Geometry check sheet. Reference: the model listing, model coordinates, mm. Face numbers are marked on the shaded views. A direction names the side the tool comes from. Coordinates: 2 decimals unless noted, no trailing zeros. Write each loop counter-clockwise with the first axis right and the second up, starting at its lowest first coordinate (ties: lowest second). Pieces come first, ordered by that corner, then holes. Notation, with made-up numbers: M 52.25,-12 L 66.25,-12 A7 cw 66.25,-3 Z; hole C 8,-24 d8. An arc over 180 degrees is marked long. Answer as a JSON object with one key per item and string values. Group by question number.
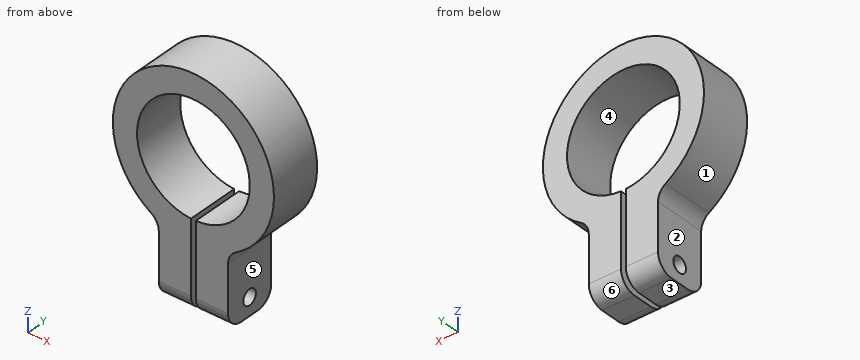
```python
from build123d import *

# Parameters (mm, degrees)
F1_DEPTH = 6.5
F2_R     = 0.95
F3_DEPTH = 25
F4_R     = 2
F5_R     = 2


with BuildPart() as f1:
    # F0 (on Front) → F1 (new body)
    with BuildSketch(Plane.XZ):
        with BuildLine():
            Line((4.29925, -18.028646), (4.29925, -9.028646))
            ThreePointArc((4.29925, -9.028646), (0, 10), (-4.29925, -9.028646))
            Line((-4.29925, -9.028646), (-4.29925, -18.028646))
            Line((-4.29925, -18.028646), (-0.29925, -18.028646))
            Line((-0.29925, -18.028646), (-0.29925, -6.993601))
            ThreePointArc((-0.29925, -6.993601), (0, 7), (0.29925, -6.993601))
            Line((0.29925, -6.993601), (0.29925, -18.028646))
            Line((0.29925, -18.028646), (4.29925, -18.028646))
        make_face()
    extrude(amount=F1_DEPTH)

    # F2 (on face) → F3 (cut)
    with BuildSketch(Plane.YZ.offset(4.29925)):
        with Locations((-3.25, -15.828646)):
            Circle(F2_R)
    extrude(amount=-F3_DEPTH, mode=Mode.SUBTRACT)

    # F4
    f4_edges = [f1.edges().sort_by_distance(p)[0] for p in [
        (2.29925, 0, -18.028646),
        (-2.29925, 0, -18.028646),
        (2.29925, -6.5, -18.028646),
        (-2.29925, -6.5, -18.028646),
    ]]
    fillet(f4_edges, radius=F4_R)

    # F5
    f5_edges = [f1.edges().sort_by_distance(p)[0] for p in [
        (4.29925, -3.25, -9.028646),
        (-4.29925, -3.25, -9.028646),
    ]]
    fillet(f5_edges, radius=F5_R)


solid = f1.part
```
1) Section check D-D (x = -6.5). Record the cut outline in (y, z), then the cut area to 3 significant figures.
2) Draft check along X on the marked faces 1, 2, 3 and 4. Enter one of: +X half, -X half, draft (parallel to the pull), parting line (faces both ways), or undercut.
3) Set-up check for the marked faces 5 and 6: record each of +Z, -Z, +X, -X, +Y, -Y from which the full face is reachable in a straight line by a thin tool's end or side.
4) Go/stop test with flat-tipped pins: pin 1 Ø3 at (y, z) = (-4, -14.5) entering from -X; pin 2 Ø2.5 at (y, z) = (-3.25, -15.83) entering from +X; pin 3 Ø3 at (y, z) = (-4, -5) entering from -X. Record where each tip stops, or that it passes through.
5) Section check C-C (z = 0). Record the cut outline in (x, y).
6) Section check B-B (x = 2). Record the cut outline in (y, z).
7) Material ranges on probe 1 along X at (y, z) = (-5, -15); probe 2 along X at (y, z) = (-4.25, 0); probe 3 along Z at (x, y) = (-0.5, -3.5), recorded low to high. Write a range as [from, to].
8) Section check A-A (y = -3.25). Record the cut outline in (x, z).
Entries:
{
 "1": {"outline": "M -6.5,-7.6 L 0,-7.6 L 0,-2.6 L -6.5,-2.6 Z; M -6.5,2.6 L 0,2.6 L 0,7.6 L -6.5,7.6 Z", "area": "65.0 mm^2"},
 "2": {"face 1": "parting line", "face 2": "-X half", "face 3": "draft", "face 4": "undercut"},
 "3": {"face 5": "-Z, +X, +Y, -Y", "face 6": "-Z, +X, -X, +Y"},
 "4": {"pin 1": "x = -4.3", "pin 2": "x = 4.3", "pin 3": "x = -9.37"},
 "5": {"outline": "M -10,-6.5 L -7,-6.5 L -7,0 L -10,0 Z; M 7,-6.5 L 10,-6.5 L 10,0 L 7,0 Z"},
 "6": {"outline": "M -6.5,-16.03 A2 ccw -4.5,-18.03 L -2,-18.03 A2 ccw 0,-16.03 L 0,-6.71 L -6.5,-6.71 Z; M -6.5,6.71 L 0,6.71 L 0,9.8 L -6.5,9.8 Z; hole C -3.25,-15.83 d1.9"},
 "7": {"probe 1": "[-4.3, -0.3], [0.3, 4.3]", "probe 2": "[-10, -7], [7, 10]", "probe 3": "[-18.03, -16.75], [-14.91, -6.98], [6.98, 9.99]"},
 "8": {"outline": "M -5.25,-8.51 A2 cw -4.3,-10.21 L -4.3,-14.88 L -0.3,-14.88 L -0.3,-6.99 A7 cw long 0.3,-6.99 L 0.3,-14.88 L 4.3,-14.88 L 4.3,-10.21 A2 cw 5.25,-8.51 A10 ccw long Z; M -4.3,-18.03 L -0.3,-18.03 L -0.3,-16.78 L -4.3,-16.78 Z; M 0.3,-18.03 L 4.3,-18.03 L 4.3,-16.78 L 0.3,-16.78 Z"}
}
